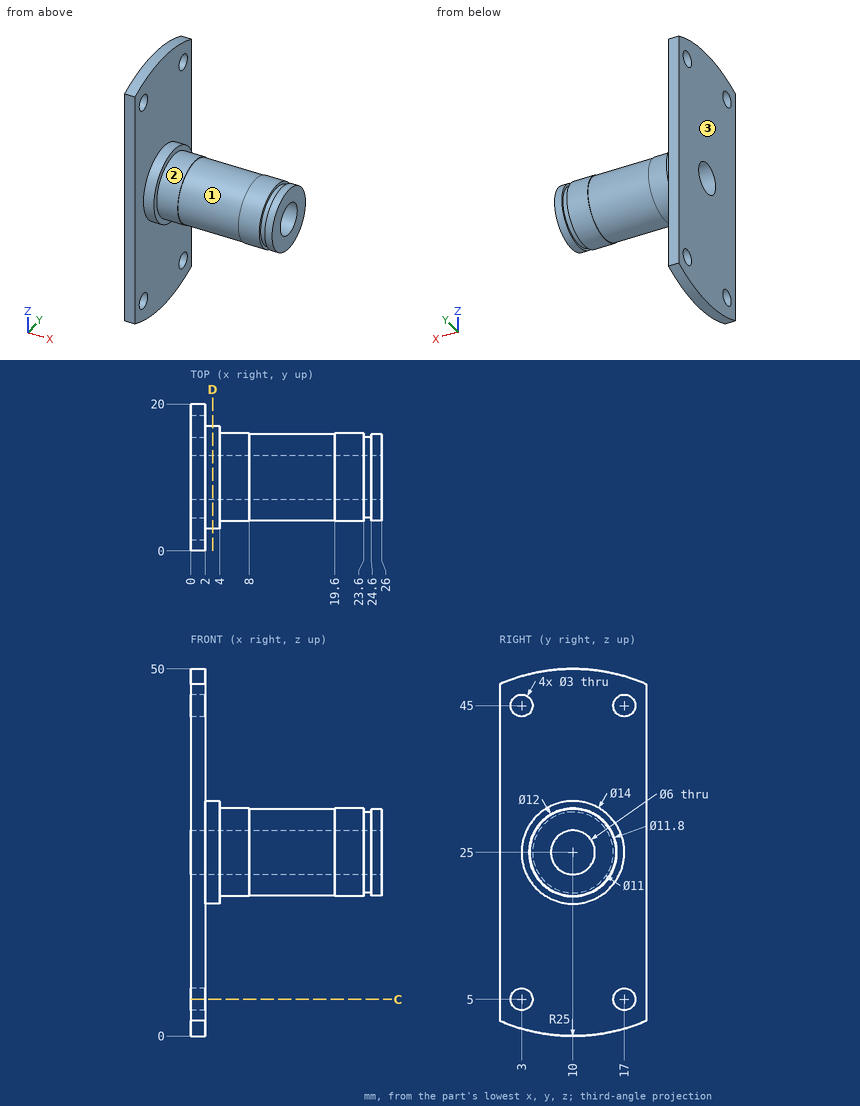
Drawing for the job (mm, zero at the part's lowest x, y, z). A direction names the side the tool comes from. Round coordinates to 2 decimals unless told otherwise and drop trailing zeros. Write each loop counter-clockwise with the first axis right and the second up, starting at its lowest first coordinate (ties: lowest second). Pieces come first, ordered by that corner, then holes. Notation, with made-up numbers: M 54,51.5 L 80,51.5 A35 ccw 80,89.5 Z; hole C -25,-0.5 d3. An arc over 180 degrees is marked long. Answer as a JSON object with one key per item and string values. Group by question number.
(1) Which spindle directions (+Z, -Z, +X, -X, +Y, -Y) get a long thin tool onto all of the face, cutting with end or side? Do the marked faces 1, 2 and 3. Say none if no direction does.
(2) Flat gauge pins, fed straight in: pin 1 (5 mm diameter, centred on x = 16.5, y = 3.5, fed in from +Z); pin 2 (3.5 mm diameter, centred on y = 17, z = 45, fed in from +X); pin 3 (8 mm diameter, centred on x = 9, z = 17.5, fed in from +Y); pin 4 (3.5 mm diameter, centred on y = 10, z = 25, fed in from -X). Where does each tip first touch, or does it go through?
(3) Drill centre lines: L1, parallel to Y at x = 0.9, z = 5; L2, parallel to Y at x = 19.25, z = 25; L3, parallel to X at y = 17, z = 7. Where is each one in solid material? Low to high.
(4) Cut at D-D (x = 3). Give the cut face in (y, z).
(5) Cut at C-C (z = 5). Give the cut face in (x, y).
Responses:
{
 "1": {"face 1": "none", "face 2": "+X", "face 3": "+Z, -Z, -X, +Y, -Y"},
 "2": {"pin 1": "stops at z = 29.34", "pin 2": "stops at x = 2", "pin 3": "stops at y = 14.78", "pin 4": "passes through"},
 "3": {"L1": "y = 0 to 1.5, 4.5 to 15.5, 18.5 to 20", "L2": "y = 4.1 to 7, 13 to 15.9", "L3": "x = 0 to 2"},
 "4": {"outline": "C 10,25 d14; hole C 10,25 d6"},
 "5": {"outline": "M 0,0 L 2,0 L 2,1.5 L 0,1.5 Z; M 0,4.5 L 2,4.5 L 2,15.5 L 0,15.5 Z; M 0,18.5 L 2,18.5 L 2,20 L 0,20 Z"}
}
